Autodesk Inventor part; units mm, degrees
ref_plane "YZ Plane" through (0, 0, 0) normal (1, 0, 0) x (0, 1, 0)
ref_plane "XZ Plane" through (0, 0, 0) normal (0, 1, 0) x (-1, 0, 0)
ref_plane "XY Plane" through (0, 0, 0) normal (0, 0, 1) x (1, 0, 0)
sketch "Sketch1" plane through (0, 0, 0) normal (1, 0, 0) x (0, 1, 0)
  line L0 (10, -1) -> (7, -1)
  line L1 (0, -1) -> (0, -4.2642) construction
  line L2 (0, -5.25) -> (3.2, -5.25)
  line L3 (3.2, -5.25) -> (3.2, -6)
  line L4 (3.2, -6) -> (10, -6)
  line L5 (10, -6) -> (10, -1)
  line L6 (10, 0) -> (0, 0) construction
  line L7 (-2, 0) -> (12, 0)
  line L8 (7, -1) -> (0, -4.2642)
  line L9 (7, -1) -> (0, -1) construction
  line L10 (0, -4.2642) -> (0, -5.25)
  point P0 (0, -4.7571)
  point P1 (5, 0)
  dimension "d2" = 6
  dimension "d3" = 5.25
  dimension "d4" = 6.8
  dimension "d9" = 3
  dimension "d10" = 155
  dimension "d11" = 1
  dimension "d12" = 10
  dimension "d13" = 5
  dimension "d16" = 3.2
revolve "Revolution1" add sketch "Sketch1" angle 360 about axis through (0, -10, 0) along (0, 1, 0)
fillet "Fillet1" radius 0.2 1 edges at (0, 3.2, 5.25)
fillet "Fillet2" radius 0.36 1 edges at (0, 0, 4.2642)
properties part number "tapon optica SiPM"
Work out the finished part from the listing and answer in its coordinate system (mm). Give positions to 0.01 mm unless a question says otherwise; leave off trailing zeros. Write each loop counter-clockwise with the first axis right and the second up, starting at its lowest first coordinate (ties: lowest second). Pieces come first, ordered by that corner, then holes. Notation, with made-up numbers: (18, 41) - (49, 41) arc R24 ccw to (49, 57) - close; hole circle Ø4 at (-15.5, -9.75). An arc over 180 degrees is marked (long way). Use one line per item in the form item = value.
1. A cutting plane is placed at C-C (y = 7.5). Write down the section's boundary in (x, z), and give its area (3 significant figures).
Filled in:
outline = circle Ø12 at (0, 0); hole circle Ø2 at (0, 0)
area = 110 mm^2
2. Determine the mould class of faces 1 (the face through (-1.37, 4.31, 1.79)), 2 (the face through (-1.6, 1.5, -5)), 3 (the face through (5, 3.2, -3)) for opening direction Z: released by +Z, released by -Z, zero draft, split by the parting line, or undercut.
Filled in:
face_1 = undercut
face_2 = split by the parting line
face_3 = zero draft
3. Each of these flat-tipped pins is pushed along its axis until it touches: pin 1 Ø6 at (x, y) = (4.5, 8) entering from -Z; pin 2 Ø2.5 at (x, z) = (0, 0) entering from -Y; pin 3 Ø3 at (x, y) = (-3, 4.5) entering from +Z. Where does it stop, or does it pass through?
Filled in:
pin_1 = -5.81
pin_2 = 6.46
pin_3 = 5.81
4. Consider L1, parallel to Z at x = 0, y = 8.95; L2, parallel to X at y = 2.25, z = 1.75. Determine where each line is inside the solid, lowest interval first.
Filled in:
L1 = -6 to -1, 1 to 6
L2 = -4.95 to -2.7, 2.7 to 4.95
5. A cutting plane is placed at B-B (x = 0). Write down the section's boundary in (y, z), and give its area (3 significant figures).
Filled in:
outline = (0, -5.25) - (3, -5.25) arc R0.2 cw to (3.2, -5.45) - (3.2, -6) - (10, -6) - (10, -1) - (7, -1) - (0.21, -4.17) arc R0.36 ccw to (0, -4.49) - close; (0, 4.49) arc R0.36 ccw to (0.21, 4.17) - (7, 1) - (10, 1) - (10, 6) - (3.2, 6) - (3.2, 5.45) arc R0.2 cw to (3, 5.25) - (0, 5.25) - close
area = 72.3 mm^2
6. A cutting plane is placed at D-D (y = 1.25). Write down the section's boundary in (x, z).
Filled in:
outline = circle Ø10.5 at (0, 0); hole circle Ø7.36 at (0, 0)
7. A cutting plane is placed at A-A (z = 0). Write down the section's boundary in (x, y), and give its area (3 significant figures).
Filled in:
outline = (-6, 3.2) - (-5.45, 3.2) arc R0.2 cw to (-5.25, 3) - (-5.25, 0) - (-4.49, 0) arc R0.36 ccw to (-4.17, 0.21) - (-1, 7) - (-1, 10) - (-6, 10) - close; (1, 7) - (4.17, 0.21) arc R0.36 ccw to (4.49, 0) - (5.25, 0) - (5.25, 3) arc R0.2 cw to (5.45, 3.2) - (6, 3.2) - (6, 10) - (1, 10) - close
area = 72.3 mm^2
